Source: three-view drawing plus pictorial views. Frame: mm from the lowest corner of the part. Round coordinates to 2 decimals unless told otherwise and drop trailing zeros. Loops run counter-clockwise (first coordinate to the right, second up) from the corner with the lowest first, then second, coordinate; pieces in that order, holes last. Notation, with made-up numbers: (-10, 62) -> (2, 62) arc R20 cw to (2, 77) -> close; hole circle Ø3 at (54, -36). An arc over 180 degrees is marked (long way). Answer in a Markdown table with one row per item. Add a question column.
Q1. Section B-B, the plane x = 8.5. Output: boundary loops of the cut face in (y, z), and give its area (3 significant figures).
Q2. Ray query, L1, parallel to X at y = 7.5, z = 1.75; L2, parallel to X at y = 18.5, z = 10.5. Return the intervals inside material, ascending. Write a range as from..to.
Q3. Pin query (flat end, axial travel): pin 1 (4 mm diameter, centred on x = 9, y = 16.5, fed in from +Z); pin 2 (2.5 mm diameter, centred on y = 8.5, z = 9, fed in from +X); pin 3 (3 mm diameter, centred on y = 18.5, z = 2, fed in from -X); pin 4 (3 mm diameter, centred on y = 14.5, z = 2.5, fed in from +X). Return the tip coordinate at first contact, or that it passes through.
Q4. Mould query, pull axis Z, two halves, no side actions, for the marked faces 1, 2 and 3. Classes: pulls with the +Z half, pulls with the -Z half, needs draft (parallel to the pull), parting line crosses it, or undercut.
Q5. Section A-A, the plane y = 5.5. Output: boundary loops of the cut face in (x, z).
Q6. Section C-C, the plane z = 10. Output: boundary loops of the cut face in (x, y), and give its area (3 significant figures).
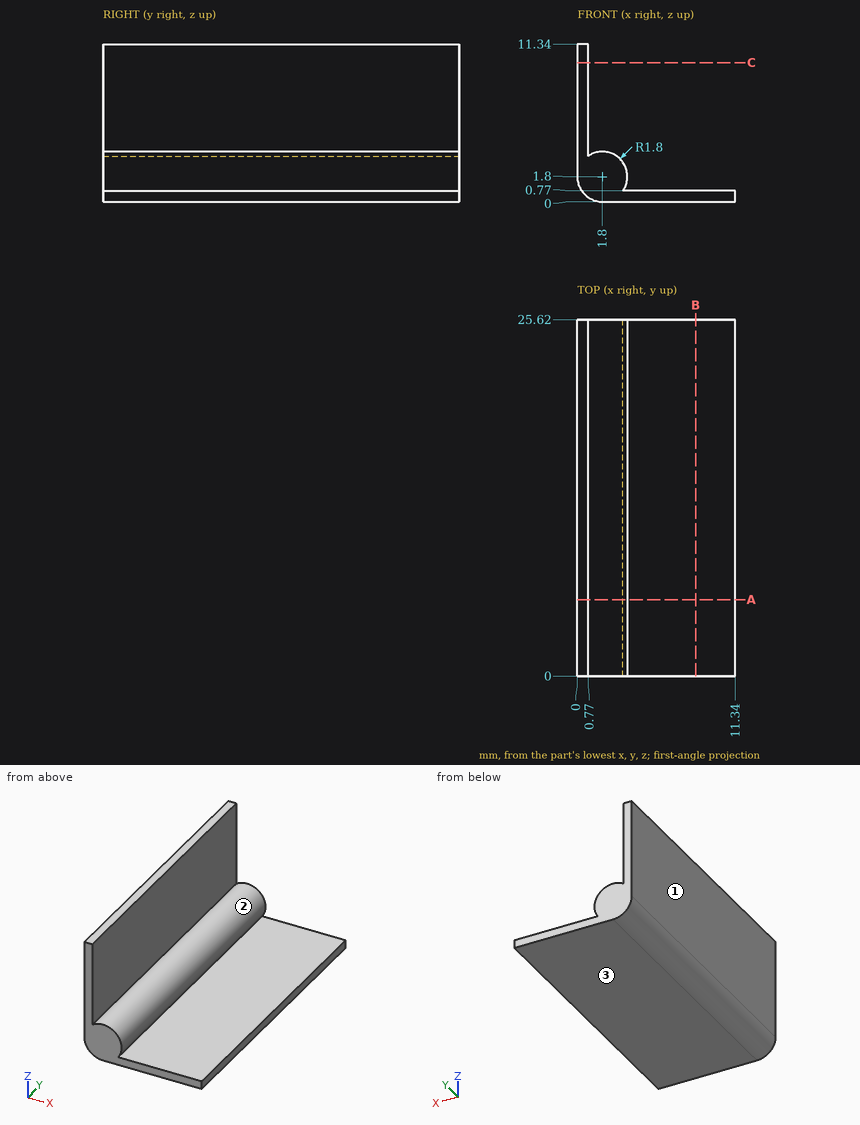
Answer block:
| question | item | result |
|---|---|---|
| 1 | outline | (0, 0) -> (25.62, 0) -> (25.62, 0.77) -> (0, 0.77) -> close |
| 1 | area | 19.7 mm^2 |
| 2 | L1 | 0..3.6 |
| 2 | L2 | 0..0.77 |
| 3 | pin 1 | z = 0.77 |
| 3 | pin 2 | x = 0.77 |
| 3 | pin 3 | x = 0 |
| 3 | pin 4 | x = 3.6 |
| 4 | face 1 | needs draft |
| 4 | face 2 | undercut |
| 4 | face 3 | pulls with the -Z half |
| 5 | outline | (0, 1.8) arc R1.8 ccw to (1.8, 0) -> (11.34, 0) -> (11.34, 0.77) -> (3.28, 0.77) arc R1.8 ccw to (0.77, 3.28) -> (0.77, 11.34) -> (0, 11.34) -> close |
| 6 | outline | (0, 0) -> (0.77, 0) -> (0.77, 25.62) -> (0, 25.62) -> close |
| 6 | area | 19.7 mm^2 |
